Geometry check sheet. Reference: the model listing, model coordinates, mm. A direction names the side the tool comes from. Coordinates: 2 decimals unless noted, no trailing zeros. Loops run counter-clockwise (first coordinate to the right, second up) from the corner with the lowest first, then second, coordinate; pieces in that order, holes last.
Solid Edge part; units mm, degrees
sketch "Sketch1" plane through (0, 0, 0) normal (0, 0, 1) x (1, 0, 0)
  line L0 (30, 105) -> (30, 30)
  line L1 (30, 30) -> (60, 30)
  line L2 (60, 30) -> (60, 105)
  line L3 (60, 105) -> (30, 105)
  line L4 (120, 30) -> (0, 30)
  line L5 (0, 30) -> (0, 0)
  line L6 (0, 0) -> (120, 0)
  line L7 (120, 0) -> (120, 30)
  line L8 (60, 0) -> (60, -30)
  line L9 (60, -30) -> (30, -30)
  line L10 (30, -30) -> (30, 0)
  line L11 (30, 0) -> (60, 0)
extrude "Protrusion1" add sketch "Sketch1" along normal blind 3
fillet "RoundMain" radius 15 8 edges at (0, 30, 1.5) (30, 105, 1.5) (60, 105, 1.5) (120, 30, 1.5) (120, 0, 1.5) (0, 0, 1.5) (60, -30, 1.5) (30, -30, 1.5)
1) Material ranges on probe 1 along X at (y, z) = (85.5, 1.65); probe 2 along Y at (x, z) = (77, 2.45); probe 3 along X at (y, z) = (97, 1.15), recorded low to high.
Data:
probe 1: x = 30 to 60
probe 2: y = 0 to 30
probe 3: x = 31.73 to 58.27
2) Section check B-B on x = 69. Record the cut outline in (y, z), and give its area (3 significant figures).
Data:
outline: (0, 0) - (30, 0) - (30, 3) - (0, 3) - close
area: 90.0 mm2
3) Access from +Z, -Z, +X, -X, +Y, -Y to the whole of each face (thin tool, end or side, straight path). Record for faces 1 (the flat face through (46, 23, 0)), 2 (the flat face through (60, -7, 1)), 3 (the flat face through (22, 0, 1)), 4 (the flat face through (23, 30, 1)), 5 (the flat face through (60, 60, 1)).
Data:
face 1: -Z, +X, -X, +Y, -Y
face 2: +Z, -Z, +X, -Y
face 3: +Z, -Z, -X, -Y
face 4: +Z, -Z, -X, +Y
face 5: +Z, -Z, +X, +Y
4) Depth check by flat-ended pin: pin 1 (1.5 mm diameter, centred on y = -4.5, z = 1, fed in from -X); pin 2 (1.5 mm diameter, centred on x = 24, z = 1.5, fed in from +Y); pin 3 (1.5 mm diameter, centred on x = 19, z = 1.5, fed in from -Y). Enter the tip coordinate at first touch or a pass-through.
Data:
pin 1: stops at x = 30
pin 2: stops at y = 30
pin 3: stops at y = 0
5) Section check C-C on y = 81. Record the cut outline in (x, z), and give its area (3 significant figures).
Data:
outline: (30, 0) - (60, 0) - (60, 3) - (30, 3) - close
area: 90.0 mm2
